```python
from build123d import *

# Parameters (mm, degrees)
F0_R     = 6.25
F1_DEPTH = 1
F2_R     = 7
F3_DEPTH = 14
F6_R     = 1.5
F7_DEPTH = 12.5


with BuildPart() as f1:
    # F0 (on Top) → F1 (new body)
    with BuildSketch(Plane.XY):
        Circle(F0_R)
    extrude(amount=-F1_DEPTH)

    # F2 (on face) → F3 (join)
    with BuildSketch(Plane(origin=(0, 0, -1), x_dir=(1, 0, 0), z_dir=(0, 0, -1))):
        Circle(F2_R)
    extrude(amount=F3_DEPTH)

    # F4 (on Right) → F5 (revolve, cut)
    with BuildSketch(Plane.YZ):
        Polygon((0, -15), (0, -1.0399731109), (-4.75, -4), (-4.75, -11.0161577418), (-6.2, -15), align=None)
    revolve(axis=Axis((0, 0, -15), (0, 0, -1)), mode=Mode.SUBTRACT)

    # F6 (on Front) → F7 (cut, symmetric)
    with BuildSketch(Plane.XZ):
        with Locations((0, -8)):
            Circle(F6_R)
    extrude(amount=F7_DEPTH, both=True, mode=Mode.SUBTRACT)


solid = f1.part
```
For this review, take the finished solid that the model builds, in its own axes (mm). A direction names the side the tool comes from. Round coordinates to 2 decimals unless told otherwise and drop trailing zeros. Order: outer loops, then holes, each group sorted by start corner. A loop starts at its lowest first (then second) coordinate and runs counter-clockwise, first axis right, second up.
Q1. Insertion check: P1, Ø4, axis at x = -4.5, z = -1.5, coming from the -Y side; P2, Ø2, axis at x = -3, z = -9, coming from the -Y side; P3, Ø2.5, axis at x = 0, z = -8, coming from the -Y side; P4, Ø4, axis at x = -4, z = -3.5, coming from the +Y side. Each pin has a flat end and moves straight along its axis. Give the tip position at first contact, or say it passes through.
Findings below:
P1: stops at y = -6.54
P2: stops at y = -6.71
P3: passes through
P4: stops at y = 6.71
Q2. We need section D-D, the plane z = -3.5. Give the boundary of the cut face in (x, y), plus the area to 3 significant figures.
Findings below:
outline: circle Ø14 at (0, 0); hole circle Ø7.9 at (0, 0)
area: 105 mm2
Q3. We need section C-C, the plane x = 1.25. State how many separate pieces and enclosed holes the cut face has, plus the area to 3 significant figures.
Findings below:
separate pieces: 3
enclosed holes: 0
area: 79.1 mm2
Q4. We need section B-B, the plane z = -8. Give the boundary of the cut face in (x, y), plus the area to 3 significant figures.
Findings below:
outline: (-1.5, -6.84) - (-1.5, -4.51) arc R4.75 cw to (-1.5, 4.51) - (-1.5, 6.84) arc R7 ccw to start; (1.5, -6.84) arc R7 ccw to (1.5, 6.84) - (1.5, 4.51) arc R4.75 cw to (1.5, -4.51) - close
area: 69.4 mm2
Q5. We need section A-A, the plane z = -10.25. Give the boundary of the cut face in (x, y), plus the area to 3 significant figures.
Findings below:
outline: circle Ø14 at (0, 0); hole circle Ø9.5 at (0, 0)
area: 83.1 mm2
Q6. Wall thickness on line 1 (X direction, y = -5.1, z = -8); line 2 (Y direction, x = -4.75, z = -13.5); line 3 (X direction, y = -5.75, z = -8): over which ranges is each line inside the solid? List them lowest first.
Findings below:
line 1: x = -4.79 to -1.5, 1.5 to 4.79
line 2: y = -5.14 to -3.07, 3.07 to 5.14
line 3: x = -3.99 to -1.5, 1.5 to 3.99
Q7. Machinability: for faces 1 (the cylindrical face through (1.819, -4.388, -7.557)), 2 (the flat face through (-3, -6, -1)), 3 (the cylindrical face through (-1.5, -5.77, -7.93)), which of the approach directions +Z, -Z, +X, -X, +Y, -Y give a long, thin tool a straight path to every point of the face, cutting with its end or side? Answer none if there is none.
Findings below:
face 1: -Z
face 2: +Z
face 3: +Y, -Y
Q8. Mouldability with a two-part tool opening along X and no side actions: class faces 4 (the flat face through (0, 0, 0)), 5 (the cylindrical face through (1.386, 5.738, -8.575)), 6 (the cylindrical face through (5.96, 1.88, -0.49)) as pulls with the +X half, pulls with the -X half, needs draft (parallel to the pull), parting line crosses it, or undercut.
Findings below:
face 4: needs draft
face 5: undercut
face 6: parting line crosses it
